Read the model definition and answer for the solid it produces. Units are mm, in the model's axes. Give positions to 0.01 mm unless a question says otherwise; leave off trailing zeros. Write each loop counter-clockwise with the first axis right and the second up, starting at its lowest first coordinate (ties: lowest second). Pieces come first, ordered by that corner, then holes.
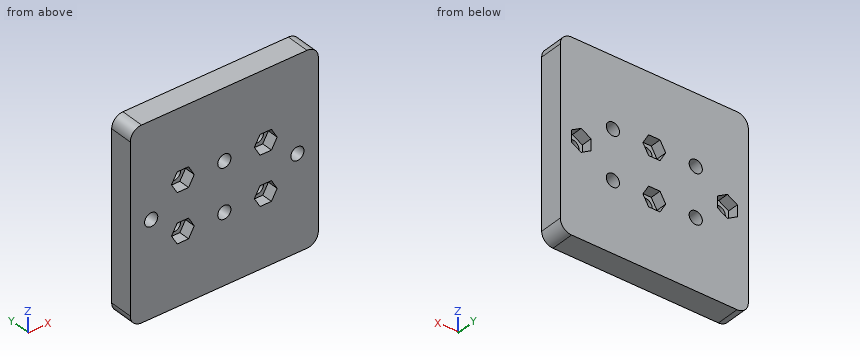
Autodesk Inventor part; units mm, degrees
ref_plane "YZ Plane" through (0, 0, 0) normal (1, 0, 0) x (0, 1, 0)
ref_plane "XZ Plane" through (0, 0, 0) normal (0, 1, 0) x (-1, 0, 0)
ref_plane "XY Plane" through (0, 0, 0) normal (0, 0, 1) x (1, 0, 0)
sketch "Boceto1" plane through (0, 0, 0) normal (0, 1, 0) x (-1, 0, 0)
  line L0 (-38.575, 38.575) -> (38.575, 38.575)
  line L1 (38.575, 38.575) -> (38.575, -38.575)
  line L2 (38.575, -38.575) -> (-38.575, -38.575)
  line L3 (-38.575, -38.575) -> (-38.575, 38.575)
  line L4 (-38.575, 38.575) -> (38.575, -38.575) construction
  line L5 (38.575, 38.575) -> (-38.575, -38.575) construction
  circle A0 centre (30, 0) radius 2.7
  circle A1 centre (-30, 0) radius 2.7
  circle A2 centre (0, 10) radius 2.7
  circle A3 centre (0, -10) radius 2.7
  point P0 (0, 0)
  dimension "d0" = 5.4
  dimension "d1" = 60
  dimension "d3" = 20
  dimension "d4" = 10
  dimension "d5" = 30
  dimension "d6" = 77.15
  dimension "d7" = 77.15
extrude "Extrusión1" add sketch "Boceto1" along normal blind 9.6
sketch "Boceto2" plane through (0, 9.6, 0) normal (0, 1, 0) x (1, 0, 0)
  circle A0 centre (-17, -10) radius 2.7
  circle A1 centre (-17, 10) radius 2.7
  circle A2 centre (17, -10) radius 2.7
  circle A3 centre (17, 10) radius 2.7
  line L0 (38.575, 38.575) -> (-38.575, 38.575)
  point P0 (0, 0)
  dimension "d10" = 5.4
  dimension "d11" = 17
  dimension "d13" = 20
  dimension "d14" = 10
  dimension "d15" = 17
extrude "Extrusión2" cut sketch "Boceto2" against normal through all
sketch "Boceto3" plane through (0, 9.6, 0) normal (0, 1, 0) x (1, 0, 0)
  circle A0 centre (-30, 0) radius 2.7
  circle A1 centre (-30, 0) radius 4.05
  line L0 (-30, 4.6765) -> (-25.95, 2.3383)
  line L1 (-25.95, 2.3383) -> (-25.95, -2.3383)
  line L2 (-25.95, -2.3383) -> (-30, -4.6765)
  line L3 (-30, -4.6765) -> (-34.05, -2.3383)
  line L4 (-34.05, -2.3383) -> (-34.05, 2.3383)
  line L5 (-34.05, 2.3383) -> (-30, 4.6765)
  circle A2 centre (0, 10) radius 2.7
  circle A3 centre (0, 10) radius 4.05
  circle A4 centre (0, -10) radius 2.7
  circle A5 centre (0, -10) radius 4.05
  circle A6 centre (30, 0) radius 2.7
  circle A7 centre (30, 0) radius 4.05
  line L6 (4.6765, 10) -> (2.3383, 5.95)
  line L7 (2.3383, 5.95) -> (-2.3383, 5.95)
  line L8 (-2.3383, 5.95) -> (-4.6765, 10)
  line L9 (-4.6765, 10) -> (-2.3383, 14.05)
  line L10 (-2.3383, 14.05) -> (2.3383, 14.05)
  line L11 (2.3383, 14.05) -> (4.6765, 10)
  line L12 (4.6765, -10) -> (2.3383, -14.05)
  line L13 (2.3383, -14.05) -> (-2.3383, -14.05)
  line L14 (-2.3383, -14.05) -> (-4.6765, -10)
  line L15 (-4.6765, -10) -> (-2.3383, -5.95)
  line L16 (-2.3383, -5.95) -> (2.3383, -5.95)
  line L17 (2.3383, -5.95) -> (4.6765, -10)
  line L18 (34.05, -2.3383) -> (30, -4.6765)
  line L19 (30, -4.6765) -> (25.95, -2.3383)
  line L20 (25.95, -2.3383) -> (25.95, 2.3383)
  line L21 (25.95, 2.3383) -> (30, 4.6765)
  line L22 (30, 4.6765) -> (34.05, 2.3383)
  line L23 (34.05, 2.3383) -> (34.05, -2.3383)
  point P0 (0, 0)
  dimension "d18" = 8.1
extrude "Extrusión3" cut sketch "Boceto3" against normal blind 4.5 contours A0 | A1 | L1 L2 A1 | A1 L0 L1 | A1 L5 L0 | L2 L3 A1 | A1 L4 L5 | L3 L4 A1 | A2 | A3 | A3 L11 L6 | A3 L10 L11 | L6 L7 A3 | A3 L9 L10 | L7 L8 A3 | A3 L8 L9 | A4 | A5 | A5 L17 L12 | A5 L16 L17 | L12 L13 A5 | A5 L15 L16 | L13 L14 A5 | A5 L14 L15 | A6 | A7 | L23 L18 A7 | A7 L22 L23 | A7 L21 L22 | L18 L19 A7 | A7 L20 L21 | L19 L20 A7
fillet "Empalme1" radius 4.635 4 edges at (-38.575, 4.8, 38.575) (38.575, 4.8, 38.575) (38.575, 4.8, -38.575) (-38.575, 4.8, -38.575)
sketch "Boceto4" plane through (0, 0, 0) normal (0, -1, 0) x (1, 0, 0)
  circle A0 centre (-17, 10) radius 2.7
  circle A1 centre (-17, 10) radius 4.05
  line L0 (-19.3383, 14.05) -> (-14.6617, 14.05)
  line L1 (-14.6617, 14.05) -> (-12.3235, 10)
  line L2 (-12.3235, 10) -> (-14.6617, 5.95)
  line L3 (-14.6617, 5.95) -> (-19.3383, 5.95)
  line L4 (-19.3383, 5.95) -> (-21.6765, 10)
  line L5 (-21.6765, 10) -> (-19.3383, 14.05)
  point P0 (0, 0)
  dimension "d22" = 8.1
extrude "Extrusión4" cut sketch "Boceto4" against normal blind 4.5 contours A0 | A1 | A1 L1 L2 | A1 L0 L1 | L2 L3 A1 | A1 L5 L0 | L3 L4 A1 | A1 L4 L5
pattern_linear "Patrón rectangular1" count 2 spacing 34 along (1, 0, 0) count 2 spacing 20 along (0, 0, -1) of "Extrusión4"
properties part number "UpperJawSupport" material "Plástico ABS"
Item 1: Section C-C (y = 3.5) is taken. Give the number of separate pieces and of enclosed holes in the cut face, and give its area (3 significant figures).
Result set:
separate pieces: 1
enclosed holes: 8
area: 5,610 mm2
Item 2: Find the intervals of material crossed by line 1 along X through (y, z) = (6.2, -10) (1 decimal); line 2 along Z through (x, y) = (0, 4) (3 decimals); line 3 along X through (y, z) = (3.65, 0) (3 decimals), in increasing order.
Result set:
line 1: x = -38.6 to -19.7, -14.3 to -4.7, 4.7 to 14.3, 19.7 to 38.6
line 2: z = -38.575 to -12.7, -7.3 to 7.3, 12.7 to 38.575
line 3: x = -38.575 to -32.7, -27.3 to 27.3, 32.7 to 38.575
Item 3: Section B-B (x = 17) is taken. Write down the section's boundary in (y, z) (3 decimals), and give its area (3 significant figures).
Result set:
outline: (0, -38.575) - (9.6, -38.575) - (9.6, -12.7) - (4.5, -12.7) - (4.5, -14.05) - (0, -14.05) - close; (0, -5.95) - (4.5, -5.95) - (4.5, -7.3) - (9.6, -7.3) - (9.6, 7.3) - (4.5, 7.3) - (4.5, 5.95) - (0, 5.95) - close; (0, 14.05) - (4.5, 14.05) - (4.5, 12.7) - (9.6, 12.7) - (9.6, 38.575) - (0, 38.575) - close
area: 613 mm2
Item 4: Section D-D (x = 28.5) is taken. Write down the section's boundary in (y, z) (1 decimal), and give its area (3 significant figures).
Result set:
outline: (0, -38.6) - (9.6, -38.6) - (9.6, -3.8) - (5.1, -3.8) - (5.1, -2.2) - (0, -2.2) - close; (0, 2.2) - (5.1, 2.2) - (5.1, 3.8) - (9.6, 3.8) - (9.6, 38.6) - (0, 38.6) - close
area: 683 mm2
Item 5: Each of these flat-tipped pins is pushed along its axis until it touches: pin 1 Ø6 at (x, z) = (0, -10) entering from +Y; pin 2 Ø3 at (x, z) = (-17, -10) entering from -Y. Where does it stop, or does it pass through?
Result set:
pin 1: stops at y = 5.1
pin 2: passes through
Item 6: Section A-A (z = 0) is taken. Write down the section's boundary in (x, y) (3 decimals), and give its area (3 significant figures).
Result set:
outline: (-38.575, 0) - (-32.7, 0) - (-32.7, 5.1) - (-34.05, 5.1) - (-34.05, 9.6) - (-38.575, 9.6) - close; (-27.3, 0) - (27.3, 0) - (27.3, 5.1) - (25.95, 5.1) - (25.95, 9.6) - (-25.95, 9.6) - (-25.95, 5.1) - (-27.3, 5.1) - close; (32.7, 0) - (38.575, 0) - (38.575, 9.6) - (34.05, 9.6) - (34.05, 5.1) - (32.7, 5.1) - close
area: 613 mm2
